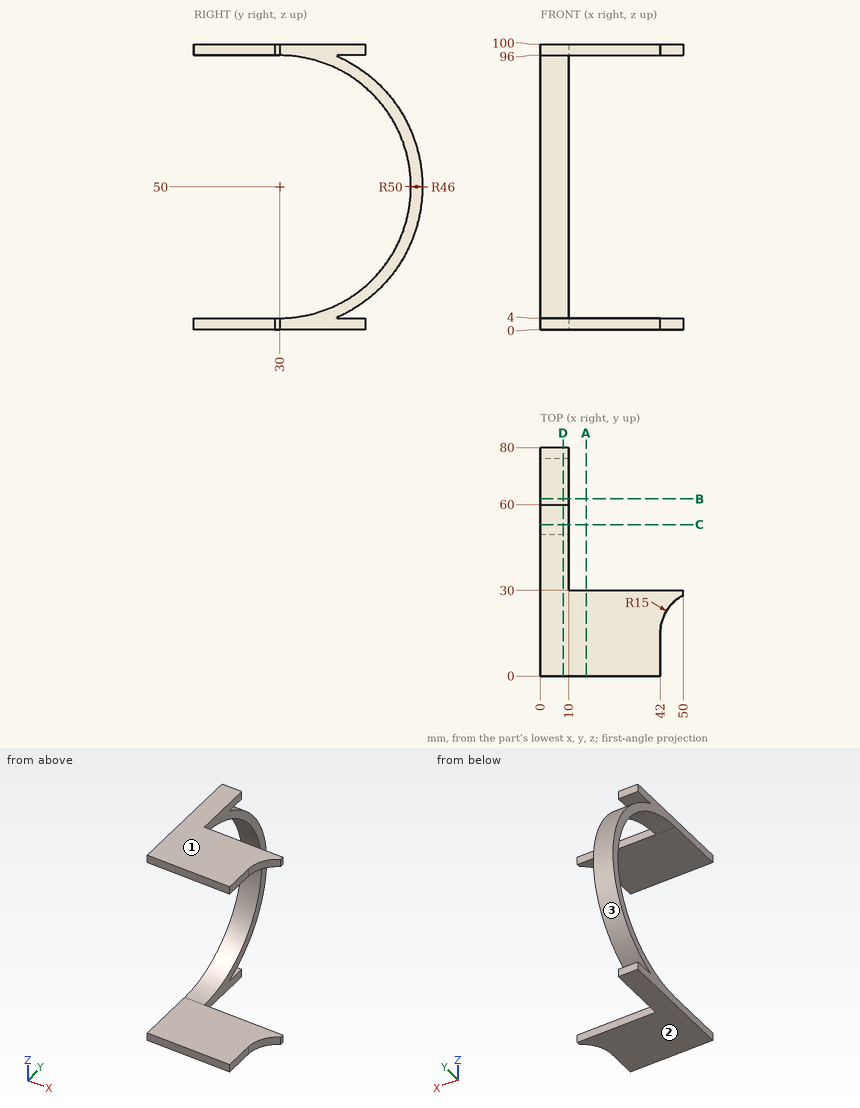
Study the drawing (mm; zero at the part's minimum x, y, z) and answer. Round coordinates to 2 decimals unless told otherwise and drop trailing zeros. Write each loop counter-clockwise with the first axis right and the second up, starting at its lowest first coordinate (ties: lowest second). Pieces come first, ordered by that corner, then holes. Notation, with made-up numbers: (33, 5) - (55, 5) arc R20 ccw to (55, 10) - close; hole circle Ø10 at (-35, 22). An arc over 180 degrees is marked (long way). Return JSON: item names as keys, results as strings. Group by question number.
Q1. The mould has two halves that part along Z. Classify the marked faces 1, 2 and 3: released by +Z, released by -Z, zero draft, split by the parting line, or undercut.
Q2. The part is cut by section D-D on x = 8. Write down the section's boundary in (y, z).
Q3. Each of these flat-tipped pins is pushed along its axis until it touches: pin 1 Ø3 at (y, z) = (4, 98) entering from +X; pin 2 Ø1.2 at (x, z) = (34.5, 99) entering from +Y; pin 3 Ø1.2 at (x, z) = (5, 98) entering from +Y. Where does it stop, or does it pass through?
Q4. The part is cut by section B-B on y = 62. Write down the section's boundary in (x, z).
Q5. Find the intervals of material crossed by L1, parallel to Z at x = 48, y = 28; L2, parallel to X at y = 76, z = 69; L3, parallel to Z at x = 9, y = 37, in increasing order.
Q6. The part is cut by section A-A on x = 16. Write down the section's boundary in (y, z).
Q7. The part is cut by section C-C on y = 53. Write down the section's boundary in (x, z), then the cut area to 3 significant figures.
Solved:
{
 "1": {"face 1": "released by +Z", "face 2": "released by -Z", "face 3": "undercut"},
 "2": {"outline": "(0, 0) - (60, 0) - (60, 4) - (49.6, 4) arc R50 ccw to (49.6, 96) - (60, 96) - (60, 100) - (0, 100) - (0, 96) - (30, 96) arc R46 cw to (30, 4) - (0, 4) - close"},
 "3": {"pin 1": "x = 42", "pin 2": "y = 30", "pin 3": "y = 60"},
 "4": {"outline": "(0, 11.58) - (10, 11.58) - (10, 16.95) - (0, 16.95) - close; (0, 83.05) - (10, 83.05) - (10, 88.42) - (0, 88.42) - close"},
 "5": {"L1": "0 to 4, 96 to 100", "L2": "0 to 10", "L3": "0 to 4.54, 95.46 to 100"},
 "6": {"outline": "(0, 0) - (30, 0) - (30, 4) - (0, 4) - close; (0, 96) - (30, 96) - (30, 100) - (0, 100) - close"},
 "7": {"outline": "(0, 0) - (10, 0) - (10, 4) - (0, 4) - close; (0, 5.6) - (10, 5.6) - (10, 10.16) - (0, 10.16) - close; (0, 89.84) - (10, 89.84) - (10, 94.4) - (0, 94.4) - close; (0, 96) - (10, 96) - (10, 100) - (0, 100) - close", "area": "171 mm²"}
}
